Build history of the part. All positions in model axes, mm. A direction names the side the tool comes from. Round coordinates to 2 decimals unless told otherwise and drop trailing zeros. Loops run counter-clockwise (first coordinate to the right, second up) from the corner with the lowest first, then second, coordinate; pieces in that order, holes last. Notation, with made-up numbers: (27, 23.25) -> (84, 23.25) arc R14 cw to (84, 33.25) -> close; hole circle Ø4 at (31.25, 48). An arc over 180 degrees is marked (long way). Put each result on its own line as item: value. Start each with the question number.
Item 1: Drill centre lines: probe 1 along Y at (x, z) = (26, -3); probe 2 along X at (y, z) = (10.5, 1.5) (3 decimals); probe 3 along Z at (x, y) = (-12, -22). Where is each one in solid material? Low to high. Write a range as [from, to].
Item 2: Tool access for faces 1 (the flat face through (-11.43, -10, 0)), 2 (the flat face through (-33, 45, -8.89)), 3 (the flat face through (-26, 48.26, 0)), 4 (the flat face through (-11.43, -33, 0)): list every direction of +Z, -Z, +X, -X, +Y, -Y with a clear straight run to the whole face (end or side of a thin tool).
Item 3: Flat gauge pins, fed straight in: pin 1 Ø19.5 at (x, y) = (-26, 52.5) entering from -Z; pin 2 Ø10 at (x, z) = (29, -3.5) entering from -Y; pin 3 Ø10 at (x, z) = (-24, -2) entering from -Y. Where does each tip first touch, or does it go through?
Item 4: Cut at A-A, the plane y = 19. List the corners of the cut face in (x, z) (3 decimals), plus the area to 3 significant figures.
Item 5: Pull direction Y, two halves, no side cores. Call faces 5 (the flat face through (0, -21, 7.62)), 6 (the flat face through (32.385, 28, 0)), 7 (the flat face through (0, -34.29, 0)), 8 (the flat face through (28, 67.31, 0)): +Y half, -Y half, draft (parallel to the pull), parting line (faces both ways), or undercut.
Item 6: Cut at C-C, the plane z = 0. List the corners of the cut face in (x, y) (1 decimal), plus the area to 3 significant figures.
Item 7: Cut at D-D, the plane y = -21.59. List the corners of the cut face in (x, z).
Item 8: Cut at B-B, the plane x = 5.5. List the corners of the cut face in (y, z), plus the area to 3 significant figures.
```python
from build123d import *

# Parameters (mm, degrees)
SKETCH1_W           = 74.93
SKETCH1_H           = 17.78
BOSS_EXTRUDE1_DEPTH = 20.32
SKETCH2_W           = 5.08
SKETCH2_H           = 39.37
BOSS_EXTRUDE2_DEPTH = 8.89
SKETCH3_W           = 17.78
SKETCH3_H           = 19.05
BOSS_EXTRUDE3_DEPTH = 8.89
SKETCH5_W           = 22.86
SKETCH5_H           = 25.4
BOSS_EXTRUDE4_DEPTH = 7.62
SKETCH6_R           = 11.1125
BOSS_EXTRUDE5_DEPTH = 25.4


with BuildPart() as part:
    # Sketch1 → Boss-Extrude1 (new, symmetric)
    with BuildSketch(Plane.XY):
        Rectangle(SKETCH1_W, SKETCH1_H)
    extrude(amount=BOSS_EXTRUDE1_DEPTH, both=True)

    # Sketch2 → Boss-Extrude2 (add, symmetric)
    with BuildSketch(Plane.XY):
        with Locations((-34.925, 28.575)):
            Rectangle(SKETCH2_W, SKETCH2_H)
        with Locations((34.925, 28.575)):
            Rectangle(SKETCH2_W, SKETCH2_H)
    extrude(amount=BOSS_EXTRUDE2_DEPTH, both=True)

    # Sketch3 → Boss-Extrude3 (add, symmetric)
    with BuildSketch(Plane.XY):
        with Locations((28.575, 57.785)):
            Rectangle(SKETCH3_W, SKETCH3_H)
        with Locations((-28.575, 57.785)):
            Rectangle(SKETCH3_W, SKETCH3_H)
    extrude(amount=BOSS_EXTRUDE3_DEPTH, both=True)

    # Sketch5 → Boss-Extrude4 (add, symmetric)
    with BuildSketch(Plane.XY):
        with Locations((0, -21.59)):
            Rectangle(SKETCH5_W, SKETCH5_H)
    extrude(amount=BOSS_EXTRUDE4_DEPTH, both=True)

    # Sketch6 → Boss-Extrude5 (add)
    with BuildSketch(Plane.ZY.offset(11.43)):
        with Locations(Location((0, -21.59, 0), (0, 0, 46.708192407))):
            Circle(SKETCH6_R)
    extrude(amount=BOSS_EXTRUDE5_DEPTH)


solid = part.part
```
Reply:
1. probe 1: y = [-8.89, 8.89], [48.26, 67.31]
1. probe 2: x = [-37.465, -32.385], [32.385, 37.465]
1. probe 3: z = [-11.1, 11.1]
2. face 1: -X
2. face 2: -Z, +X, -X, +Y
2. face 3: +Z, -Z
2. face 4: -X, -Y
3. pin 1: stops at z = -8.89
3. pin 2: stops at y = -8.89
3. pin 3: stops at y = -32.7
4. outline: (-37.465, -8.89) -> (-32.385, -8.89) -> (-32.385, 8.89) -> (-37.465, 8.89) -> close; (32.385, -8.89) -> (37.465, -8.89) -> (37.465, 8.89) -> (32.385, 8.89) -> close
4. area: 181 mm^2
5. face 5: draft
5. face 6: undercut
5. face 7: -Y half
5. face 8: +Y half
6. outline: (-37.5, -8.9) -> (-11.4, -8.9) -> (-11.4, -10.5) -> (-36.8, -10.5) -> (-36.8, -32.7) -> (-11.4, -32.7) -> (-11.4, -34.3) -> (11.4, -34.3) -> (11.4, -8.9) -> (37.5, -8.9) -> (37.5, 67.3) -> (19.7, 67.3) -> (19.7, 48.3) -> (32.4, 48.3) -> (32.4, 8.9) -> (-32.4, 8.9) -> (-32.4, 48.3) -> (-19.7, 48.3) -> (-19.7, 67.3) -> (-37.5, 67.3) -> close
6. area: 3,550 mm^2
7. outline: (-36.83, -11.11) -> (-11.43, -11.11) -> (-11.43, -7.62) -> (11.43, -7.62) -> (11.43, 7.62) -> (-11.43, 7.62) -> (-11.43, 11.11) -> (-36.83, 11.11) -> close
8. outline: (-34.29, -7.62) -> (-8.89, -7.62) -> (-8.89, -20.32) -> (8.89, -20.32) -> (8.89, 20.32) -> (-8.89, 20.32) -> (-8.89, 7.62) -> (-34.29, 7.62) -> close
8. area: 1,110 mm^2
